from build123d import *

# Parameters (mm, degrees)
SKETCH1_R           = 50
BOSS_EXTRUDE1_DEPTH = 30
CIRPATTERN1_COUNT   = 8


# Read off the part's stored shape, not the designer's step: Sketch-Pattern1
with BuildPart() as part:
    # Sketch1 → Boss-Extrude1 (new body)
    with BuildSketch(Plane(origin=(0, 0, 0), x_dir=(1, 0, 0), z_dir=(0, 1, 0))):
        with Locations(Location((0, 0, 0), (0, 0, 270))):
            Circle(SKETCH1_R)
    extrude(amount=BOSS_EXTRUDE1_DEPTH)

    # Sketch5 → CBORE for M5 Hex Head Cap Screw1 (revolve, cut)
    with BuildSketch(Plane(origin=(0, 30, -40), x_dir=(0, 0, 1), z_dir=(1, 0, 0))):
        Polygon((0, 0), (0, 20), (2.5, 18.497848452), (2.5, 10), (5, 10), (5, 0), align=None)
    cbore_for_m5_hex_head_cap_screw1 = revolve(axis=Axis((0, 36.35, -40), (0, -1, 0)), mode=Mode.SUBTRACT)

    # CirPattern1: CBORE for M5 Hex Head Cap Screw1 ×8 about axis
    cirpattern1_axis = Axis((0, 0, 0), (0, 1, 0))
    for i in range(1, CIRPATTERN1_COUNT):
        add(cbore_for_m5_hex_head_cap_screw1.rotate(cirpattern1_axis, i * 360 / CIRPATTERN1_COUNT), mode=Mode.SUBTRACT)

    # Sketch6 → Hole Wizard 950 (revolve, cut)
    with BuildSketch(Plane(origin=(-18.945239219, 30, 5.62940246), x_dir=(0, 0, 1), z_dir=(1, 0, 0))):
        Polygon((0, 0), (0, 20), (0.9, 19.459225443), (0.9, 1.1), (3.3475, 1.1), (3.3475, 0), align=None)
    hole_wizard_950 = revolve(axis=Axis((-18.945239219, 36.35, 5.62940246), (0, -1, 0)), mode=Mode.SUBTRACT)

    # Sketch-Pattern1 outline → Sketch-Pattern1 (revolve, cut)
    with BuildSketch(Plane(origin=(-23.333134216, 0, 10.487429063), x_dir=(1, 0, 0), z_dir=(0, 0, 1))):
        Polygon((3.3475, 30), (0, 30), (0, 10), (0.9, 10.540774557), (0.9, 28.9), (3.3475, 28.9), align=None)
    revolve(axis=Axis((-23.333134216, 0, 10.487429063), (0, 1, 0)), mode=Mode.SUBTRACT)

    # Sketch-Pattern2: Hole Wizard 950 at 6 more places
    with Locations((0.112884, 0, -23.151681), (-4.729973, 0, -17.769404), (3.49498, 0, -18.713251), (5.247838, 0, -26.533698), (-4.729973, 0, -28.691063), (6.191685, 0, -30.848427)):
        add(hole_wizard_950, mode=Mode.SUBTRACT)


solid = part.part
Verification items for the finished model (mm, model axes). A direction names the side the tool comes from. Give positions to 0.01 mm unless a question says otherwise; leave off trailing zeros. Loops run counter-clockwise (first coordinate to the right, second up) from the corner with the lowest first, then second, coordinate; pieces in that order, holes last.
1) Depth check by flat-ended pin: pin 1 Ø4 at (x, z) = (-15.45, -13.08) entering from +Y; pin 2 Ø4 at (x, z) = (-10, -34) entering from -Y; pin 3 Ø2 at (x, y) = (12, 6) entering from +Z (3 decimals); pin 4 Ø8 at (x, y) = (-24, 14) entering from +Z. Enter the tip coordinate at first touch or a pass-through.
2) Sectioned sample at B-B, the plane z = 32. Enter the section's corners in (x, y).
3) Sectioned sample at A-A, the plane y = 13.5. Count the separate pieces of the cut face and the enclosed holes in it, then the cut area to 3 significant figures.
4) Sectioned sample at D-D, the plane z = 16.5. Enter the section's corners in (x, y).
5) Draft check along X on faces 1 (the cylindrical face through (15.02, 14.79, 47.69)), 2 (the cylindrical face through (28.5, 25.07, -33.28)), 3 (the flat face through (1, 0, -1)). Enter one of: pulls with the +X half, pulls with the -X half, needs draft (parallel to the pull), parting line crosses it, or undercut.
6) Sectioned sample at C-C, the plane x = 20. Enter the section's corners in (y, z).
7) Thickness scan on line 1 along Y through (x, z) = (-32.5, 27); line 2 along X through (y, z) = (18.25, 30.5); line 3 along X through (y, z) = (10.5, 39.5). Record the ranges inside material, lowest first.
8) Set-up check for faces 4 (the cylindrical face through (0, 25, 45)), 5 (the flat face through (1, 30, -1)): record each of +Z, -Z, +X, -X, +Y, -Y from which the full face is reachable in a straight line by a thin tool's end or side.
Answers:
1. pin 1: stops at y = 28.9
1. pin 2: stops at y = 0
1. pin 3: stops at z = 48.775
1. pin 4: stops at z = 45.83
2. outline: (-38.42, 0) - (38.42, 0) - (38.42, 30) - (31.63, 30) - (31.63, 20) - (24.94, 20) - (24.94, 30) - (-24.94, 30) - (-24.94, 20) - (-31.63, 20) - (-31.63, 30) - (-38.42, 30) - close
3. separate pieces: 1
3. enclosed holes: 16
3. area: 7,680 mm2
4. outline: (-47.2, 0) - (47.2, 0) - (47.2, 30) - (-47.2, 30) - close
5. face 1: parting line crosses it
5. face 2: undercut
5. face 3: needs draft
6. outline: (0, -45.83) - (30, -45.83) - (30, 45.83) - (0, 45.83) - close
7. line 1: y = 0 to 20
7. line 2: x = -39.62 to -29.44, -27.13 to 27.13, 29.44 to 39.62
7. line 3: x = -30.66 to -0.67, 0.67 to 30.66
8. face 4: +Y
8. face 5: +Z, -Z, +X, -X, +Y
